Could you check a few things on this model? Use its own coordinates, in mm. Face numbers are marked on the shaded views. A direction names the side the tool comes from. Round coordinates to 2 decimals unless told otherwise and drop trailing zeros. Loops run counter-clockwise (first coordinate to the right, second up) from the corner with the lowest first, then second, coordinate; pieces in that order, holes last. Notation, with made-up numbers: (61.5, -8) -> (81.5, -8) arc R25 cw to (81.5, 25) -> close; hole circle Ø3 at (19.5, 13). An arc over 180 degrees is marked (long way). One line per item, written item: value.
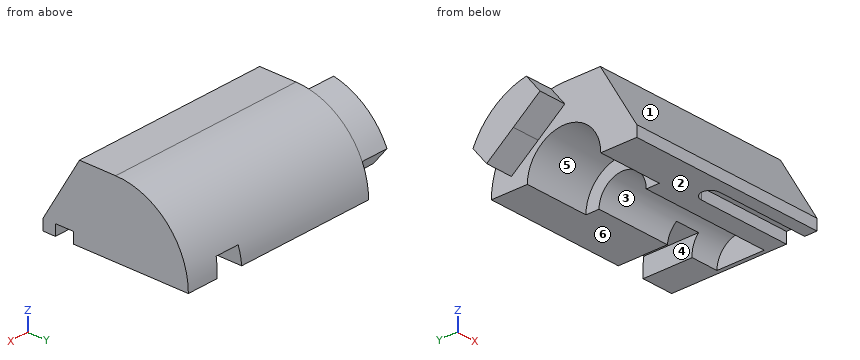
from build123d import *

# Parameters (mm, degrees)
BOSS_EXTRU_1_DEPTH      = 240
ESQUISSE2_R             = 28.575
ENL_V_MAT_EXTRU_1_DEPTH = 235
ESQUISSE3_R             = 44.45
ENL_V_MAT_EXTRU_2_DEPTH = 78
ENL_V_MAT_EXTRU_4_DEPTH = 13
BOSS_EXTRU_2_START      = -33
BOSS_EXTRU_2_DEPTH      = 33
ENL_V_MAT_EXTRU_5_DEPTH = 100


with BuildPart() as part:
    # Esquisse1 → Boss.-Extru.1 (new body)
    with BuildSketch(Plane(origin=(0, 0, 0), x_dir=(0, 0, -1), z_dir=(1, 0, 0))):
        with BuildLine():
            Line((0, 0), (0, 88))
            ThreePointArc((0, 88), (-62.225396744, 62.225396744), (-88, 0))
            Line((-88, 0), (-88, -43.853430349))
            Line((-88, -43.853430349), (-13, -88))
            Line((-13, -88), (0, -88))
            Line((0, -88), (0, 0))
        make_face()
    extrude(amount=BOSS_EXTRU_1_DEPTH)

    # Esquisse2 → Enlèv. mat.-Extru.1 (cut)
    with BuildSketch(Plane(origin=(0, 0, 0), x_dir=(0, 0, -1), z_dir=(1, 0, 0))):
        Circle(ESQUISSE2_R)
    extrude(amount=ENL_V_MAT_EXTRU_1_DEPTH, mode=Mode.SUBTRACT)

    # Esquisse3 → Enlèv. mat.-Extru.2 (cut)
    with BuildSketch(Plane(origin=(0, 0, 0), x_dir=(0, 0, -1), z_dir=(1, 0, 0))):
        Circle(ESQUISSE3_R)
    extrude(amount=ENL_V_MAT_EXTRU_2_DEPTH, mode=Mode.SUBTRACT)

    # Esquisse5 → Enlèv. mat.-Extru.4 (cut)
    with BuildSketch(Plane.XY):
        with BuildLine():
            ThreePointArc((127, -73), (116, -62), (127, -51))
            Line((127, -51), (240, -51))
            Line((240, -51), (240, -73))
            Line((240, -73), (127, -73))
        make_face()
    extrude(amount=ENL_V_MAT_EXTRU_4_DEPTH, mode=Mode.SUBTRACT)

    # Esquisse6 → Boss.-Extru.2 (add)
    with BuildSketch(Plane(origin=(0, 0, 0), x_dir=(0, 0, -1), z_dir=(1, 0, 0)).offset(BOSS_EXTRU_2_START)):
        with BuildLine():
            Line((-65.430668922, -0.909705656), (-40.188548434, 31.398735242))
            Line((-40.188548434, 31.398735242), (-14.946427946, 63.707176139))
            Line((-14.946427946, 63.707176139), (-36.116548227, 80.247086827))
            ThreePointArc((-36.116548227, 80.247086827), (-69.344946317, 54.178209829), (-86.600789204, 15.630205031))
            Line((-86.600789204, 15.630205031), (-65.430668922, -0.909705656))
        make_face()
    extrude(amount=BOSS_EXTRU_2_DEPTH)

    # Esquisse7 → Enlèv. mat.-Extru.5 (cut)
    with BuildSketch(Plane(origin=(0, 0, 0), x_dir=(1, 0, 0), z_dir=(0, 1, 0))):
        Polygon((202, 0), (169, 0), (170.857438953, -21.230624387), (200.142561047, -21.230624387), align=None)
    extrude(amount=ENL_V_MAT_EXTRU_5_DEPTH, mode=Mode.SUBTRACT)


solid = part.part
(1) If we section it at B-B, the plane z = 8.5: Please give me the cut outline in (x, y), then the cut area to 3 significant figures.
Recorded:
outline: (0, -88) -> (240, -88) -> (240, -73) -> (127, -73) arc R11 cw to (127, -51) -> (240, -51) -> (240, 87.59) -> (201.26, 87.59) -> (201.26, 27.28) -> (235, 27.28) -> (235, -27.28) -> (78, -27.28) -> (78, -43.63) -> (0, -43.63) -> close; (0, 43.63) -> (78, 43.63) -> (78, 27.28) -> (169.74, 27.28) -> (169.74, 87.59) -> (0, 87.59) -> close
area: 22,200 mm²
(2) I'm going to push flat-ended pins straight in: pin 1 Ø10 at (y, z) = (-52, 65) entering from -X; pin 2 Ø2 at (x, y) = (186, 3.5) entering from -Z; pin 3 Ø10.5 at (x, z) = (160.5, 8) entering from +Y. Where does each tip first touch, or does it pass through?
Recorded:
pin 1: x = 0
pin 2: z = 28.22
pin 3: y = 87.96
(3) If we section it at A-A, the plane x = 180: Please give me the cut outline in (y, z) (3 decimals).
Recorded:
outline: (-88, 0) -> (-73, 0) -> (-73, 13) -> (-51, 13) -> (-51, 0) -> (-28.575, 0) arc R28.575 cw to (19.126, 21.231) -> (85.401, 21.231) arc R88 ccw to (0, 88) -> (-43.853, 88) -> (-88, 13) -> close
(4) If we section it at C-C, the plane x = 92.5: Please give me the cut outline in (y, z) (3 decimals).
Recorded:
outline: (-88, 0) -> (-28.575, 0) arc R28.575 cw to (28.575, 0) -> (88, 0) arc R88 ccw to (0, 88) -> (-43.853, 88) -> (-88, 13) -> close
(5) If we section it at D-D, the plane y = -59.5: Please give me the cut outline in (x, z).
Recorded:
outline: (0, 0) -> (116.29, 0) -> (116.29, 13) -> (240, 13) -> (240, 61.42) -> (0, 61.42) -> close
(6) If I drill on L1, parallel to Y at x = 9, z = 5.5; L2, parallel to X at y = 68.5, z = 4.5; L3, parallel to X at y = 4, z = 15.5, over which ranges is the centre line in solid material (lowest first)?
Recorded:
L1: -88 to -44.11, 44.11 to 87.83
L2: 0 to 169.39, 201.61 to 240
L3: 235 to 240
(7) For the marked faces 4, 5 and 6, which set-ups out of +Z, -Z, +X, -X, +Y, -Y let a thin tool reach every point of the face, with its end or its side?
Recorded:
face 4: -Z, +Y
face 5: -Z, -X
face 6: -Z, +X, -X, +Y, -Y
(8) Thinking about a two-plate mould opening in Y: for the marked faces 1, 2 and 3, which applies, released by +Y, released by -Y, zero draft, split by the parting line, or undercut?
Recorded:
face 1: released by -Y
face 2: zero draft
face 3: undercut
